Geometry check sheet. Reference: drawing and pictorial views, mm from the part's lowest x, y, z. A direction names the side the tool comes from. Give positions to 0.01 mm unless a question says otherwise; leave off trailing zeros. Write each loop counter-clockwise with the first axis right and the second up, starting at its lowest first coordinate (ties: lowest second). Pieces come first, ordered by that corner, then holes.
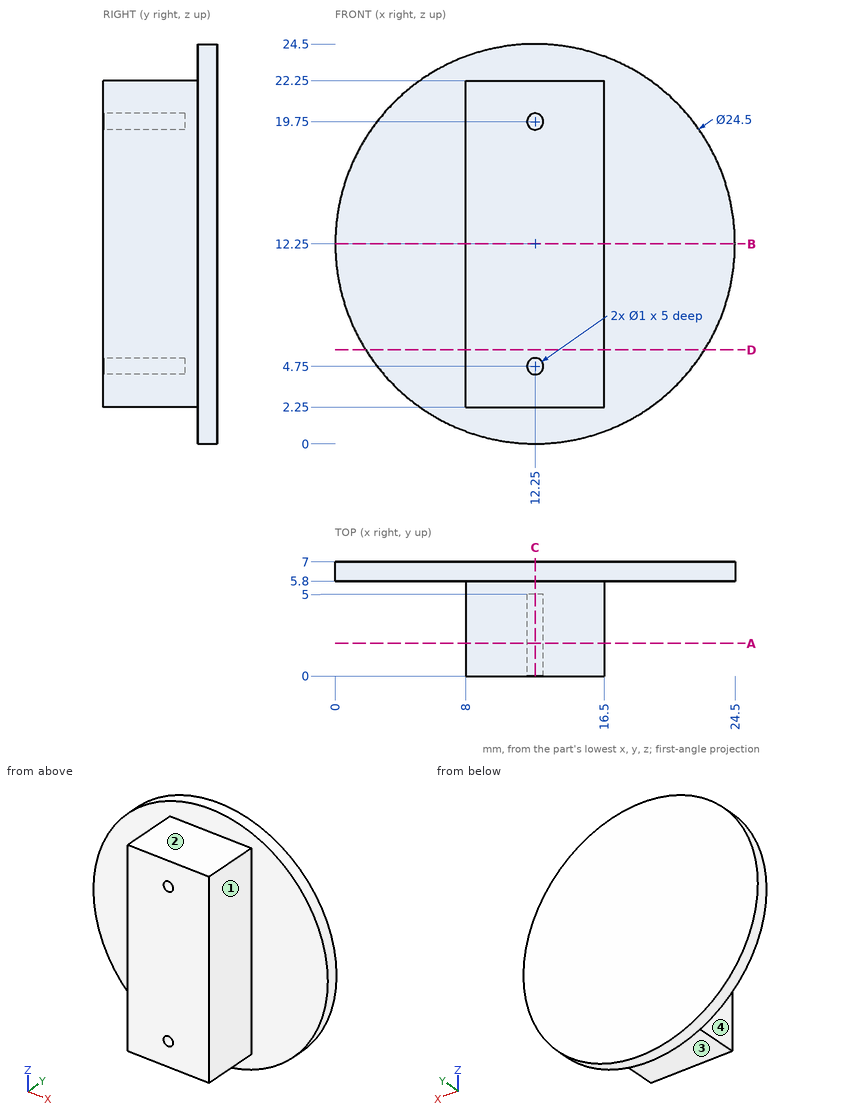
Item 1: Sectioned sample at B-B on z = 12.25. Record the cut outline in (x, y), then the cut area to 3 significant figures.
Answer key:
outline: (0, 5.8) - (8, 5.8) - (8, 0) - (16.5, 0) - (16.5, 5.8) - (24.5, 5.8) - (24.5, 7) - (0, 7) - close
area: 78.7 mm2
Item 2: Set-up check for the marked faces 1, 2, 3 and 4: record each of +Z, -Z, +X, -X, +Y, -Y from which the full face is reachable in a straight line by a thin tool's end or side.
Answer key:
face 1: +Z, -Z, +X, -Y
face 2: +Z, +X, -X, -Y
face 3: -Z, +X, -X, -Y
face 4: +Z, -Z, -X, -Y
Item 3: Sectioned sample at D-D on z = 5.75. Record the cut outline in (x, y), then the cut area to 3 significant figures.
Answer key:
outline: (1.87, 5.8) - (8, 5.8) - (8, 0) - (16.5, 0) - (16.5, 5.8) - (22.63, 5.8) - (22.63, 7) - (1.87, 7) - close
area: 74.2 mm2
Item 4: Depth check by flat-ended pin: pin 1 (1.5 mm diameter, centred on x = 5.5, y = 4, fed in from +Z); pin 2 (3 mm diameter, centred on x = 14, y = 4, fed in from +Z); pin 3 (4 mm diameter, centred on x = 14, y = 3, fed in from -Z). Enter the tip coordinate at first touch or a pass-through.
Answer key:
pin 1: passes through
pin 2: stops at z = 22.25
pin 3: stops at z = 2.25
Item 5: Sectioned sample at A-A on y = 2. Record the cut outline in (x, z).
Answer key:
outline: (8, 2.25) - (16.5, 2.25) - (16.5, 22.25) - (8, 22.25) - close; hole circle Ø1 at (12.25, 4.75); hole circle Ø1 at (12.25, 19.75)
Item 6: Sectioned sample at C-C on x = 12.25. Record the cut outline in (y, z), then the cut area to 3 significant figures.
Answer key:
outline: (0, 2.25) - (5.8, 2.25) - (5.8, 0) - (7, 0) - (7, 24.5) - (5.8, 24.5) - (5.8, 22.25) - (0, 22.25) - (0, 20.25) - (5, 20.25) - (5, 19.25) - (0, 19.25) - (0, 5.25) - (5, 5.25) - (5, 4.25) - (0, 4.25) - close
area: 135 mm2
Item 7: Scan lines: line 1 along Z through (x, y) = (12.25, 2.5); line 2 along X through (y, z) = (3.15, 19.75); line 3 along X through (y, z) = (4.25, 8). Record each from-to range of solid material in increasing order.
Answer key:
line 1: z = 2.25 to 4.25, 5.25 to 19.25, 20.25 to 22.25
line 2: x = 8 to 11.75, 12.75 to 16.5
line 3: x = 8 to 16.5
